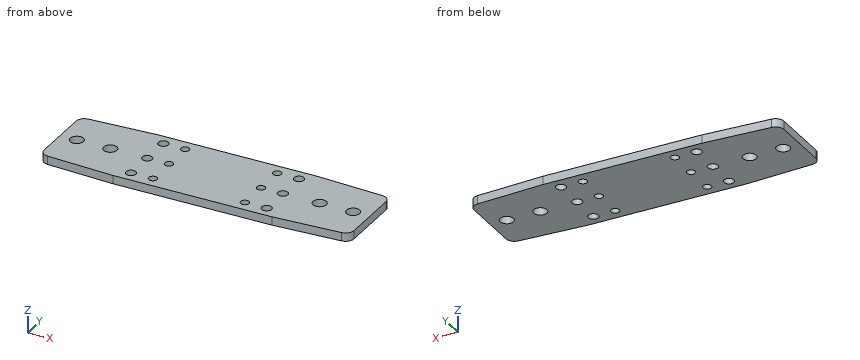
from build123d import *

# Parameters (mm, degrees)
SKETCH1_R           = 4
SKETCH1_R_2         = 2.5
SKETCH1_R_3         = 3
BOSS_EXTRUDE1_DEPTH = 5
FILLET1_R           = 5


with BuildPart() as part:
    # Sketch1 → Boss-Extrude1 (new body)
    with BuildSketch(Plane.XY):
        Polygon((95, 0), (0, 0), (-45, -2.5), (-45, -47.5), (0, -50), (95, -50), (140, -47.5), (140, -2.5), align=None)
        with Locations((-35, -25)):
            Circle(SKETCH1_R, mode=Mode.SUBTRACT)
        with Locations((-15, -25)):
            Circle(SKETCH1_R, mode=Mode.SUBTRACT)
        with Locations((75, -43)):
            Circle(SKETCH1_R_2, mode=Mode.SUBTRACT)
        with Locations((75, -7)):
            Circle(SKETCH1_R_2, mode=Mode.SUBTRACT)
        with Locations((110, -25)):
            Circle(SKETCH1_R, mode=Mode.SUBTRACT)
        with Locations((130, -25)):
            Circle(SKETCH1_R, mode=Mode.SUBTRACT)
        with Locations((20, -25)):
            Circle(SKETCH1_R_2, mode=Mode.SUBTRACT)
        with Locations((75, -25)):
            Circle(SKETCH1_R_2, mode=Mode.SUBTRACT)
        with Locations((7, -25)):
            Circle(SKETCH1_R_3, mode=Mode.SUBTRACT)
        with Locations((88, -25)):
            Circle(SKETCH1_R_3, mode=Mode.SUBTRACT)
        with Locations((20, -7)):
            Circle(SKETCH1_R_2, mode=Mode.SUBTRACT)
        with Locations((20, -43)):
            Circle(SKETCH1_R_2, mode=Mode.SUBTRACT)
        with BuildLine():
            ThreePointArc((7, -40), (4, -43), (7, -46))
            ThreePointArc((7, -46), (10, -43), (7, -40))
        make_face(mode=Mode.SUBTRACT)
        with BuildLine():
            ThreePointArc((88, -46), (91, -43), (88, -40))
            ThreePointArc((88, -40), (85, -43), (88, -46))
        make_face(mode=Mode.SUBTRACT)
        with BuildLine():
            ThreePointArc((88, -10), (91, -7), (88, -4))
            ThreePointArc((88, -4), (85, -7), (88, -10))
        make_face(mode=Mode.SUBTRACT)
        with BuildLine():
            ThreePointArc((7, -10), (10, -7), (7, -4))
            ThreePointArc((7, -4), (4, -7), (7, -10))
        make_face(mode=Mode.SUBTRACT)
    extrude(amount=BOSS_EXTRUDE1_DEPTH)

    # Fillet1
    fillet1_edges = [part.edges().sort_by_distance(p)[0] for p in [
        (140, -2.5, 2.5),
        (140, -47.5, 2.5),
        (-45, -47.5, 2.5),
        (-45, -2.5, 2.5),
    ]]
    fillet(fillet1_edges, radius=FILLET1_R)


solid = part.part
The listing builds one solid part. Answer for the finished solid, in the listing's coordinates (mm). Give positions to 0.01 mm unless a question says otherwise; leave off trailing zeros. Loops run counter-clockwise (first coordinate to the right, second up) from the corner with the lowest first, then second, coordinate; pieces in that order, holes last.
Item 1: A cutting plane is placed at A-A (x = 20). Give the vertices of the cut face in (y, z).
Derived:
outline: (-50, 0) - (-45.5, 0) - (-45.5, 5) - (-50, 5) - close; (-40.5, 0) - (-27.5, 0) - (-27.5, 5) - (-40.5, 5) - close; (-22.5, 0) - (-9.5, 0) - (-9.5, 5) - (-22.5, 5) - close; (-4.5, 0) - (0, 0) - (0, 5) - (-4.5, 5) - close
Item 2: Find the intervals of material crossed by line 1 along Y through (x, z) = (75, 3.05); line 2 along Y through (x, z) = (88, 2.65); line 3 along X through (y, z) = (-5, 0.7), in increasing order.
Derived:
line 1: y = -50 to -45.5, -40.5 to -27.5, -22.5 to -9.5, -4.5 to 0
line 2: y = -50 to -46, -40 to -28, -22 to -10, -4 to 0
line 3: x = -44.48 to 4.76, 9.24 to 18.5, 21.5 to 73.5, 76.5 to 85.76, 90.24 to 139.48
Item 3: A cutting plane is placed at D-D (x = 110). Give the vertices of the cut face in (y, z).
Derived:
outline: (-49.17, 0) - (-29, 0) - (-29, 5) - (-49.17, 5) - close; (-21, 0) - (-0.83, 0) - (-0.83, 5) - (-21, 5) - close
Item 4: This flat-tipped pin is pushed along its axis until it touches: pin 1 Ø6.5 at (x, y) = (-35, -25) entering from +Z. Where does it stop, or does it pass through?
Derived:
pin 1: passes through
Item 5: A cutting plane is placed at B-B (z = 4). Give the number of separate pieces and of enclosed holes in the cut face, then the cut area to 3 significant figures.
Derived:
separate pieces: 1
enclosed holes: 16
area: 8,520 mm2
